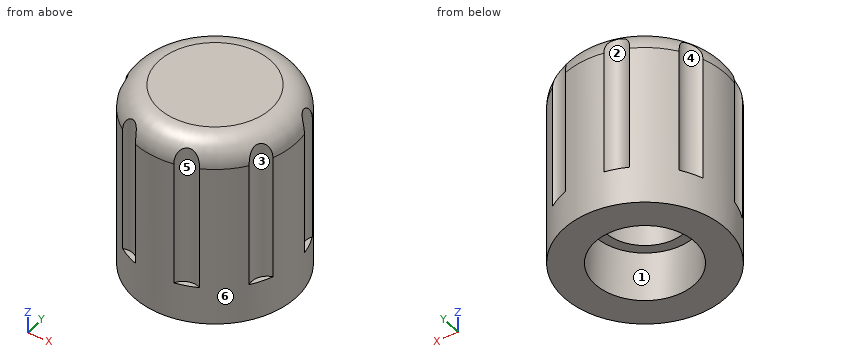
from build123d import *

# Parameters (mm, degrees)
CYLINDER_R         = 6.5
CYLINDER_DEPTH     = 15
CYLINDER001_R      = 3.2
CYLINDER001_DEPTH  = 13
BOX_W              = 2
BOX_H              = 7.5
BOX_DEPTH          = 7
FILLET_R           = 2
CYLINDER002_R      = 1.25
CYLINDER002_DEPTH  = 12
POLARPATTERN_COUNT = 8
CYLINDER003_R      = 4
CYLINDER003_DEPTH  = 4


with BuildPart() as part:
    # Cylinder → Cylinder (join)
    with BuildSketch(Plane.XY):
        Circle(CYLINDER_R)
    extrude(amount=CYLINDER_DEPTH)

    # Cylinder001 → Cylinder001 (cut)
    with BuildSketch(Plane(origin=(0, 0, 13), x_dir=(1, 0, 0), z_dir=(0, 0, -1))):
        Circle(CYLINDER001_R)
    extrude(amount=CYLINDER001_DEPTH, mode=Mode.SUBTRACT)

    # Box → Box (join)
    with BuildSketch(Plane(origin=(1.5, 3.75, 14), x_dir=(1, 0, 0), z_dir=(0, 0, -1))):
        with Locations((1, 3.75)):
            Rectangle(BOX_W, BOX_H)
    extrude(amount=BOX_DEPTH)

    # Fillet
    fillet_edges = [part.edges().sort_by_distance(p)[0] for p in [
        (-6.5, 0, 15),
    ]]
    fillet(fillet_edges, radius=FILLET_R)

    # Cylinder002 → Cylinder002 (cut)
    with BuildSketch(Plane(origin=(-6.5, 3.35, 3), x_dir=(1, 0, 0), z_dir=(0, 0, 1))):
        Circle(CYLINDER002_R)
    cylinder002 = extrude(amount=CYLINDER002_DEPTH, mode=Mode.SUBTRACT)

    # PolarPattern: Cylinder002 ×8 about axis
    polarpattern_axis = Axis((0, 0, 0), (0, 0, 1))
    for i in range(1, POLARPATTERN_COUNT):
        add(cylinder002.rotate(polarpattern_axis, i * 360 / POLARPATTERN_COUNT), mode=Mode.SUBTRACT)

    # Cylinder003 → Cylinder003 (cut)
    with BuildSketch(Plane(origin=(0, 0, 4), x_dir=(1, 0, 0), z_dir=(0, 0, -1))):
        Circle(CYLINDER003_R)
    extrude(amount=CYLINDER003_DEPTH, mode=Mode.SUBTRACT)


solid = part.part
The model under review builds one solid part; all positions refer to its coordinate system, in mm. Face numbers are marked on the shaded views. A direction names the side the tool comes from. Give positions to 0.01 mm unless a question says otherwise; leave off trailing zeros. Loops run counter-clockwise (first coordinate to the right, second up) from the corner with the lowest first, then second, coordinate; pieces in that order, holes last. Notation, with made-up numbers: (62, 69.5) -> (71, 69.5) arc R15 cw to (71, 90.5) -> close; hole circle Ø3 at (22, 60.5). An arc over 180 degrees is marked (long way). Answer as a JSON object with one key per item and string values. Group by question number.
Q1. Take a section at C-C (y = 0). Write out the cut boundary in (x, z).
Q2. Take a section at A-A (x = 0). Write out the cut boundary in (y, z).
Q3. Tool access review of the marked faces 1, 2 and 3: name each direction out of +Z, -Z, +X, -X, +Y, -Y from which nothing blocks a thin tool from reaching the whole face with its end or side.
Q4. Insertion check: pin 1 (0.7 mm diameter, centred on x = -2.5, y = -5.5, fed in from +Z); pin 2 (7.5 mm diameter, centred on x = 0, y = 0, fed in from -Z); pin 3 (4 mm diameter, centred on y = -2.5, z = 10, fed in from +X). Each pin has a flat end and moves straight along its axis. Give the tip position at first contact, or say it passes through.
Q5. Wall thickness on line 1 along Y through (x, z) = (0, 6.75); line 2 along X through (y, z) = (0, 1.9): over which ranges is each line inside the solid? List them lowest first.
Q6. Draft analysis for pull direction Y (two halves, no side actions). For the marked faces 4, 5 and 6, state which applies: pulls with the +Y half, pulls with the -Y half, needs draft (parallel to the pull), parting line crosses it, or undercut.
Answer below:
{
 "1": {"outline": "(-6.5, 0) -> (-4, 0) -> (-4, 4) -> (-3.2, 4) -> (-3.2, 13) -> (1.5, 13) -> (1.5, 7) -> (3.2, 7) -> (3.2, 4) -> (4, 4) -> (4, 0) -> (6.5, 0) -> (6.5, 13) arc R2 ccw to (4.5, 15) -> (-4.5, 15) arc R2 ccw to (-6.5, 13) -> close"},
 "2": {"outline": "(-6.5, 0) -> (-4, 0) -> (-4, 4) -> (-3.2, 4) -> (-3.2, 13) -> (3.2, 13) -> (3.2, 4) -> (4, 4) -> (4, 0) -> (6.5, 0) -> (6.5, 13) arc R2 ccw to (4.5, 15) -> (-4.5, 15) arc R2 ccw to (-6.5, 13) -> close"},
 "3": {"face 1": "-Z", "face 2": "+Z, +Y", "face 3": "+Z, +X"},
 "4": {"pin 1": "stops at z = 14.61", "pin 2": "stops at z = 4", "pin 3": "stops at x = 6.48"},
 "5": {"line 1": "y = -6.5 to -3.2, 3.2 to 6.5", "line 2": "x = -6.5 to -4, 4 to 6.5"},
 "6": {"face 4": "undercut", "face 5": "pulls with the -Y half", "face 6": "parting line crosses it"}
}
